Verification items for the finished model (mm, model axes). A direction names the side the tool comes from. Round coordinates to 2 decimals unless told otherwise and drop trailing zeros. Order: outer loops, then holes, each group sorted by start corner. A loop starts at its lowest first (then second) coordinate and runs counter-clockwise, first axis right, second up. Notation, with made-up numbers: (62, 73) -> (109, 73) arc R28 ccw to (109, 109) -> close; hole circle Ø11 at (-22, 47). An arc over 180 degrees is marked (long way). Answer in a Markdown table with one row per item. Add a question column.
Autodesk Inventor part; units mm, degrees
ref_plane "YZ Plane" through (0, 0, 0) normal (1, 0, 0) x (0, 1, 0)
ref_plane "XZ Plane" through (0, 0, 0) normal (0, 1, 0) x (-1, 0, 0)
ref_plane "XY Plane" through (0, 0, 0) normal (0, 0, 1) x (1, 0, 0)
sketch "Sketch1" plane through (0, 0, 0) normal (0, 0, 1) x (1, 0, 0)
  line L0 (-7.2739, -1.4271) -> (7.2739, -1.4271)
  line L1 (7.2739, -1.4271) -> (7.2739, 1.4271)
  line L2 (7.2739, 1.4271) -> (-7.2739, 1.4271)
  line L3 (-7.2739, 1.4271) -> (-7.2739, -1.4271)
  line L4 (-7.2739, -1.4271) -> (7.2739, 1.4271) construction
  line L5 (7.2739, -1.4271) -> (-7.2739, 1.4271) construction
  line L6 (9.525, 3.6783) -> (-9.525, 3.6783)
  line L7 (-9.525, 3.6783) -> (-9.525, 6.4723)
  line L8 (-9.525, 6.4723) -> (9.525, 6.4723)
  line L9 (9.525, 6.4723) -> (9.525, 3.6783)
  line L10 (9.525, 3.6783) -> (-9.525, 6.4723) construction
  line L11 (-9.525, 3.6783) -> (9.525, 6.4723) construction
  line L12 (-7.2739, 1.4271) -> (-9.525, 3.6783)
  line L13 (7.2739, 1.4271) -> (9.525, 3.6783)
  line L14 (-10.922, 5.0753) -> (-8.1026, 7.8947)
  line L15 (-10.922, 5.0753) -> (-6.9348, 5.0753) construction
  line L16 (-10.922, 5.0753) -> (-9.525, 3.6783)
  line L17 (10.922, 5.0753) -> (8.1026, 7.8947)
  line L18 (9.525, 3.6783) -> (10.922, 5.0753)
  line L19 (-8.1026, 7.8947) -> (8.1026, 7.8947)
  line L20 (-19.05, -1.4271) -> (19.05, -1.4271)
  line L21 (19.05, -1.4271) -> (19.05, 15.8839)
  line L22 (19.05, 15.8839) -> (-19.05, 15.8839)
  line L23 (-19.05, 15.8839) -> (-19.05, -1.4271)
  point P0 (0, 0)
  point P1 (0, 5.0753)
  point P2 (0, -1.4271)
  dimension "d0" = 135
  dimension "d1" = 135
  dimension "d2" = 19.05
  dimension "d3" = 2.794
  dimension "d4" = 45
  dimension "d5" = 4.2164
  dimension "d6" = 90
  dimension "d7" = 90
  dimension "d8" = 9.3218
  dimension "d9" = 38.1
extrude "Extrusion1" add sketch "Sketch1" against normal blind 177.8 contours L20 L23 L22 L21 L1 L13 L18 L17 L19 L14 L16 L12 L3
sketch "Sketch2" plane through (0, 0, -177.8) normal (0, 0, -1) x (-1, 0, 0)
  arc A0 (19.05, 29.7163) -> (-19.05, 29.7163) centre (0, 29.7163) ccw
  line L0 (19.05, -1.4271) -> (19.05, 15.8839)
  line L1 (19.05, 15.8839) -> (19.05, -1.4271)
  line L2 (19.05, 15.8839) -> (19.05, 29.7163)
  line L3 (-19.05, -1.4271) -> (-19.05, 15.8839)
  line L4 (-19.05, 15.8839) -> (-19.05, 29.7163)
  line L5 (19.05, 15.8839) -> (-19.05, 15.8839)
  point P0 (0, 0)
extrude "Extrusion2" add sketch "Sketch2" against normal blind 50.8
sketch "Sketch3" plane through (0, 0, -177.8) normal (0, 0, -1) x (-1, 0, 0)
  arc A0 (19.05, 29.7163) -> (-19.05, 29.7163) centre (0, 29.7163) ccw
  point P0 (0, 0)
hole "Hole1" at (0, 29.7163, -177.8) direction (0, 0, 1) diameter 21.6 end through all
fillet "Fillet1" radius 3.175 2 edges at (-19.05, 15.8839, -63.5) (19.05, 15.8839, -63.5)
sketch "Sketch4" plane through (0, 0, 0) normal (0, 0, 1) x (1, 0, 0)
  line L0 (-84.0587, 46.9015) -> (30.6415, 46.9015)
  line L1 (30.6415, 46.9015) -> (30.6415, -6.8679)
  line L2 (30.6415, -6.8679) -> (-84.0587, -6.8679)
  line L3 (-84.0587, -6.8679) -> (-84.0587, 46.9015)
  line L4 (-84.0587, 46.9015) -> (30.6415, -6.8679) construction
  line L5 (30.6415, 46.9015) -> (-84.0587, -6.8679) construction
  point P0 (0, 0)
  point P1 (-26.7086, 20.0168)
extrude "Extrusion3" cut sketch "Sketch4" against normal blind 50.8
properties part number "Laser mount 5 inches"
1) Draft check along Y on faces 1 (the face through (13, -1.427, -113)), 2 (the face through (-18.145, 14.929, -89.433)), 3 (the face through (10, 6, -113)). Enter one of: +Y half, -Y half, draft (parallel to the pull), parting line (faces both ways), or undercut.
2) Cross-section at C-C, the plane z = -104. Record the boundary of the cut face in (x, y) (3 decimals).
3) Thickness scan on L1, parallel to Y at x = 0, z = -142.5; L2, parallel to Y at x = 15.5, z = -64.5; L3, parallel to Z at x = 12.5, y = 24. Record the ranges inside material, lowest first. Write a range as [from, to].
4) Depth check by flat-ended pin: P1, Ø9.5, axis at x = -5, z = -96.5, coming from the +Y side; P2, Ø13, axis at x = 0, z = -102.5, coming from the -Y side; P3, Ø4, axis at y = 39.5, z = -164.5, coming from the -X side. Enter the tip coordinate at first touch or a pass-through.
5) Cross-section at A-A, the plane x = 0. Record the boundary of the cut face in (y, z), and give its area (3 significant figures).
6) Cross-section at D-D, the plane y = 43. Record the boundary of the cut face in (x, z).
7) Tool access check on faces 4 (the face through (0, 15.884, -88)), 5 (the face through (7.274, 0, -113)), 6 (the face through (-10, 6, -113)). Record the directions out of +Z, -Z, +X, -X, +Y, -Y that give a thin tool (end or side, any length) a straight path to the whole face; none if there is none.
8) Cross-section at B-B, the plane z = -153. Record the boundary of the cut face in (x, y) (3 decimals), and give its area (3 significant figures).
Results below:
| question | item | result |
|---|---|---|
| 1 | face 1 | -Y half |
| 1 | face 2 | +Y half |
| 1 | face 3 | undercut |
| 2 | outline | (-19.05, -1.427) -> (-7.274, -1.427) -> (-7.274, 1.427) -> (-9.525, 3.678) -> (-10.922, 5.075) -> (-8.103, 7.895) -> (8.103, 7.895) -> (10.922, 5.075) -> (9.525, 3.678) -> (7.274, 1.427) -> (7.274, -1.427) -> (19.05, -1.427) -> (19.05, 12.709) arc R3.175 ccw to (15.875, 15.884) -> (-15.875, 15.884) arc R3.175 ccw to (-19.05, 12.709) -> close |
| 3 | L1 | [7.89, 18.92], [40.52, 48.77] |
| 3 | L2 | [-1.43, 15.88] |
| 3 | L3 | [-177.8, -127] |
| 4 | P1 | y = 15.88 |
| 4 | P2 | y = 7.89 |
| 4 | P3 | x = -17.39 |
| 5 | outline | (7.89, -177.8) -> (18.92, -177.8) -> (18.92, -127) -> (15.88, -127) -> (15.88, -50.8) -> (7.89, -50.8) -> close; (40.52, -177.8) -> (48.77, -177.8) -> (48.77, -127) -> (40.52, -127) -> close |
| 5 | area | 1,590 mm² |
| 6 | outline | (-13.65, -177.8) -> (13.65, -177.8) -> (13.65, -127) -> (-13.65, -127) -> close |
| 7 | face 4 | +Z, +X, -X, +Y |
| 7 | face 5 | +Z, -Z, -Y |
| 7 | face 6 | +Z, -Z |
| 8 | outline | (-19.05, -1.427) -> (-7.274, -1.427) -> (-7.274, 1.427) -> (-9.525, 3.678) -> (-10.922, 5.075) -> (-8.103, 7.895) -> (8.103, 7.895) -> (10.922, 5.075) -> (9.525, 3.678) -> (7.274, 1.427) -> (7.274, -1.427) -> (19.05, -1.427) -> (19.05, 29.716) arc R19.05 ccw to (-19.05, 29.716) -> close; hole circle Ø21.6 at (0, 29.716) |
| 8 | area | 1,230 mm² |
